Answer from the drawing. Dimensions are ordinates in mm from the lowest x, y and z of the part. A direction names the side the tool comes from. Round coordinates to 2 decimals unless told otherwise and drop trailing zeros. Loops run counter-clockwise (first coordinate to the right, second up) from the corner with the lowest first, then second, coordinate; pieces in that order, holes last. Notation, with made-up numbers: M 82.25,89.5 L 87.25,89.5 A28 cw 87.25,125.5 Z; hole C -16,68 d10. An arc over 180 degrees is marked long. One line per item, written item: value.
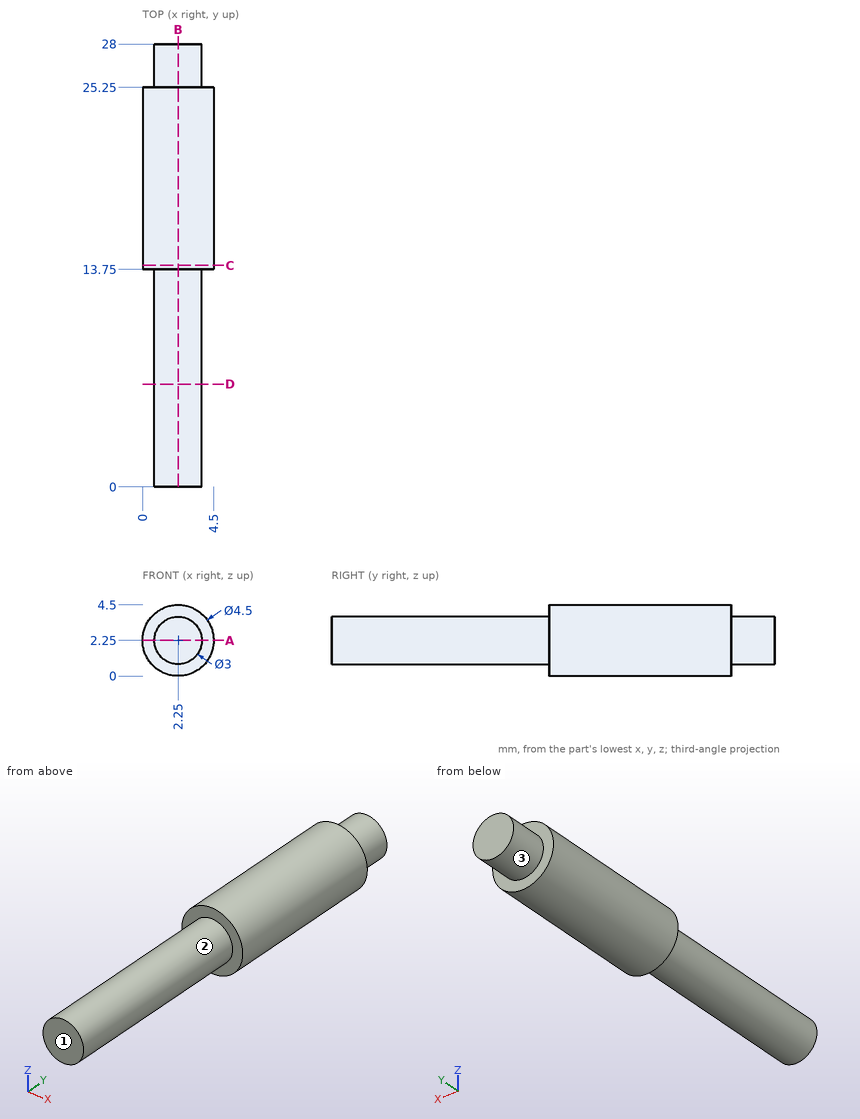
1) Find the intervals of material crossed by probe 1 along Y at (x, z) = (1.6, 0.75); probe 2 along Z at (x, y) = (1.8, 10); probe 3 along Z at (x, y) = (1.45, 18), in increasing order. Write a range as from..to.
Check values:
probe 1: 13.75..25.25
probe 2: 0.82..3.68
probe 3: 0.15..4.35
2) Find section B-B (x = 2.25). Give the vertices of the cut face in (y, z).
Check values:
outline: M 0,0.75 L 13.75,0.75 L 13.75,0 L 25.25,0 L 25.25,0.75 L 28,0.75 L 28,3.75 L 25.25,3.75 L 25.25,4.5 L 13.75,4.5 L 13.75,3.75 L 0,3.75 Z
3) Find section C-C (y = 14). Give the vertices of the cut face in (x, z), then the cut area to 3 significant figures.
Check values:
outline: C 2.25,2.25 d4.5
area: 15.9 mm2
4) Find section A-A (z = 2.25). Give the vertices of the cut face in (x, y).
Check values:
outline: M 0,13.75 L 0.75,13.75 L 0.75,0 L 3.75,0 L 3.75,13.75 L 4.5,13.75 L 4.5,25.25 L 3.75,25.25 L 3.75,28 L 0.75,28 L 0.75,25.25 L 0,25.25 Z
5) For the marked faces 1, 2 and 3, determine the directions among +Z, -Z, +X, -X, +Y, -Y from which every point of the face is accessible in a straight line to the end or side of a thin tool.
Check values:
face 1: +Z, -Z, +X, -X, -Y
face 2: -Y
face 3: +Y
6) Find section D-D (y = 6.5). Give the vertices of the cut face in (x, z).
Check values:
outline: C 2.25,2.25 d3
7) Each of these flat-tipped pins is pushed along its axis until it touches: pin 1 (1.5 mm diameter, centred on y = 16.5, z = 1.5, fed in from -X); pin 2 (1 mm diameter, centred on y = 14.5, z = 3, fed in from +X); pin 3 (1.5 mm diameter, centred on y = 4, z = 1, fed in from +X). Where does it stop, or does it pass through?
Check values:
pin 1: x = 0
pin 2: x = 4.49
pin 3: x = 3.66
